The model under review builds one solid part; all positions refer to its coordinate system, in mm. Face numbers are marked on the shaded views. A direction names the side the tool comes from. Round coordinates to 2 decimals unless told otherwise and drop trailing zeros. Write each loop counter-clockwise with the first axis right and the second up, starting at its lowest first coordinate (ties: lowest second). Pieces come first, ordered by that corner, then holes. Notation, with made-up numbers: M -28,-5 L -13,-5 A21 ccw -13,29 Z; hole C 22.5,2.5 d7. An arc over 180 degrees is marked long. Write item = value, one per line. Start each with the question number.
Item 1: Tool access review of the marked faces 1, 2 and 3: name each direction out of +Z, -Z, +X, -X, +Y, -Y from which nothing blocks a thin tool from reaching the whole face with its end or side.
Item 2: Take a section at C-C, the plane z = 0. Give the boundary of the cut face in (x, y), plus the area to 3 significant figures.
Item 3: Take a section at A-A, the plane x = 0. Give the boundary of the cut face in (y, z), plus the area to 3 significant figures.
Item 4: To check wall thickness, follow line 1 along Y through (x, z) = (-1.25, 9.5); line 2 along Y through (x, z) = (4, 7); line 3 along Z through (x, y) = (4.75, -0.25). State the ranges of each line that lie inside material, in increasing order.
Item 5: For pin 1 Ø11 at (x, z) = (0, -6) entering from +Y; pin 2 Ø2 at (y, z) = (-2.5, 10) entering from -X; pin 3 Ø2 at (x, z) = (3.5, 24) entering from +Y, all flat-tipped, find the tip position at first contact; note any pin that passes through.
Item 6: Take a section at B-B, the plane y = -2. Give the boundary of the cut face in (x, z), plus the area to 3 significant figures.
Item 7: The part is to be moulded in two halves that separate along Z. For the marked faces 4, 5, 6 and 7, say which applies: +Z half, -Z half, draft (parallel to the pull), parting line (faces both ways), or undercut.
Item 8: Take a section at D-D, the plane y = 1. Give the boundary of the cut face in (x, z), plus the area to 3 significant figures.
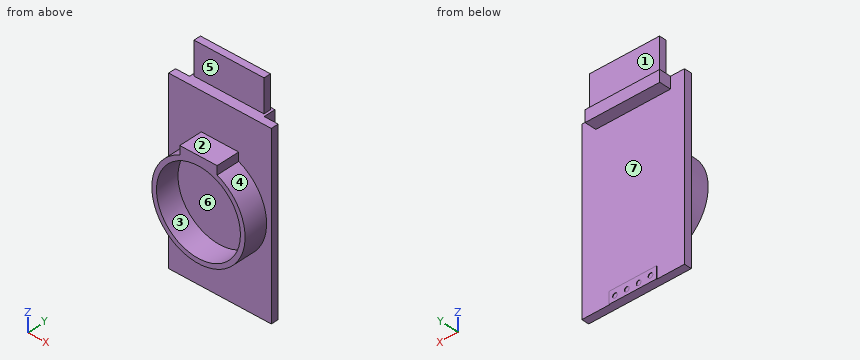
Autodesk Inventor part; units mm, degrees
ref_plane "YZ Plane" through (0, 0, 0) normal (1, 0, 0) x (0, 1, 0)
ref_plane "XZ Plane" through (0, 0, 0) normal (0, 1, 0) x (-1, 0, 0)
ref_plane "XY Plane" through (0, 0, 0) normal (0, 0, 1) x (1, 0, 0)
sketch "Sketch1" plane through (0, 0, 0) normal (0, 1, 0) x (-1, 0, 0)
  line L0 (11, -19) -> (-11, -19)
  line L1 (-11, -19) -> (-11, 19)
  line L2 (-11, 19) -> (11, 19)
  line L3 (11, 19) -> (11, -19)
  line L4 (11, -19) -> (-11, 19) construction
  line L5 (-11, -19) -> (11, 19) construction
  point P0 (0, 0)
  dimension "d0" = 22
  dimension "d1" = 38
extrude "Extrusion1" add sketch "Sketch1" along normal blind 1.6
sketch "Sketch2" plane through (0, 0, 0) normal (0, -1, 0) x (1, 0, 0)
  circle A0 centre (0, 0) radius 10
  circle A1 centre (0, 0) radius 9
  line L0 (-4, 9) -> (-4, 9)
  line L1 (-4, 9) -> (-4, 11)
  line L2 (-4, 11) -> (4, 11)
  line L3 (4, 11) -> (4, 9)
  point P0 (-4, 9.1652)
  point P1 (4, 9.1652)
  dimension "d4" = 20
  dimension "d7" = 18
  dimension "d8" = 8
  dimension "d9" = 2
  dimension "d10" = 0
extrude "Extrusion2" add sketch "Sketch2" along normal blind 5
sketch "Sketch3" plane through (0, 1.6, 0) normal (0, 1, 0) x (1, 0, 0)
  line L0 (-11, -19) -> (11, -19)
  line L1 (-8, -19) -> (8, -19)
  line L2 (8, -19) -> (8, -16.5)
  line L3 (8, -16.5) -> (-8, -16.5)
  line L4 (-8, -16.5) -> (-8, -19)
  line L5 (-11, 19) -> (-11, -19)
  line L6 (11, -19) -> (11, 19)
  point P0 (0, 0)
  dimension "d11" = 2.5
  dimension "d12" = 3
  dimension "d13" = 3
extrude "Extrusion3" add sketch "Sketch3" along normal blind 2.5
sketch "Sketch4" plane through (0, 1.6, 0) normal (0, 1, 0) x (1, 0, 0)
  line L0 (11, 19) -> (-11, 19)
  line L1 (-5.0746, 19) -> (5.08, 19)
  line L2 (5.08, 19) -> (5.08, 16.46)
  line L3 (5.08, 16.46) -> (-5.0746, 16.46)
  line L4 (-5.0746, 16.46) -> (-5.0746, 19)
  line L5 (-11, 19) -> (-11, -19)
  line L6 (11, -19) -> (11, 19)
  circle A0 centre (-3.8046, 17.73) radius 0.5
  circle A1 centre (-1.27, 17.8958) radius 0.5
  circle A2 centre (1.27, 17.8958) radius 0.5
  circle A3 centre (3.81, 17.8958) radius 0.5
  point P0 (0, 0)
  point P1 (0.0027, 19)
  point P2 (0, 19)
  dimension "d16" = 2.54
  dimension "d19" = 1
  dimension "d20" = 1
  dimension "d21" = 1
  dimension "d22" = 1
  dimension "d23" = 2.54
  dimension "d24" = 2.54
  dimension "d25" = 2.54
  dimension "d26" = 1.27
  dimension "d27" = 1.27
  dimension "d29" = 1.27
  dimension "d30" = 1.27
extrude "Extrusion4" add sketch "Sketch4" along normal blind 0.1
sketch "Sketch5" plane through (-11, 0, 19) normal (0, 0, 1) x (1, 0, 0)
  line L0 (3.5, 3.6) -> (18.5, 3.6)
  line L1 (18.5, 3.6) -> (18.5, 2.1)
  line L2 (18.5, 2.1) -> (3.5, 2.1)
  line L3 (3.5, 2.1) -> (3.5, 3.6)
  line L4 (3, 4.1) -> (19, 4.1)
  line L5 (3, 1.6) -> (3, 4.1)
  line L6 (19, 1.6) -> (19, 4.1)
  line L7 (0, 1.6) -> (3, 1.6)
  point P0 (11, 0)
  dimension "d35" = 0.5
  dimension "d36" = 0.5
  dimension "d37" = 0.5
  dimension "d38" = 0.5
extrude "Extrusion5" add sketch "Sketch5" along normal blind 7
equation "\"d13\" = d12"
properties part number "ZS042" material "PC/ABS Plastic"
Response values:
q1.face_1 = +Z, +X, -X, +Y
q1.face_2 = +Z, +X, -X, -Y
q1.face_3 = -Y
q2.outline = M -11,0 L -10,0 L -10,-5 L -9,-5 L -9,0 L 9,0 L 9,-5 L 10,-5 L 10,0 L 11,0 L 11,1.6 L -11,1.6 Z
q2.area = 45.2 mm2
q3.outline = M -5,-10 L 0,-10 L 0,-19 L 1.7,-19 L 1.7,-16.46 L 1.6,-16.46 L 1.6,16.5 L 4.1,16.5 L 4.1,19 L 3.6,19 L 3.6,26 L 2.1,26 L 2.1,19 L 0,19 L 0,11 L -5,11 L -5,9 L 0,9 L 0,-9 L -5,-9 Z
q3.area = 92.8 mm2
q4.line_1 = -5 to 1.6
q4.line_2 = 0 to 1.6
q4.line_3 = -8.8 to -7.64, 7.64 to 8.8
q5.pin_1 = 1.6
q5.pin_2 = -4.36
q5.pin_3 = 3.6
q6.outline = M -4,9.17 A10 ccw long 4,9.17 L 4,11 L -4,11 Z; hole C 0,0 d18
q6.area = 69.9 mm2
q7.face_4 = parting line
q7.face_5 = draft
q7.face_6 = undercut
q7.face_7 = undercut
q8.outline = M -11,-19 L 11,-19 L 11,19 L -11,19 Z
q8.area = 836 mm2
